Verification items for the finished model (mm, model axes). A direction names the side the tool comes from. Coordinates: 2 decimals unless noted, no trailing zeros. Write each loop counter-clockwise with the first axis right and the second up, starting at its lowest first coordinate (ties: lowest second). Pieces come first, ordered by that corner, then holes. Notation, with made-up numbers: (10.25, 7) -> (50.25, 7) arc R26 cw to (50.25, 39) -> close; hole circle Ø2 at (23, 50). An arc over 180 degrees is marked (long way). Answer in a Markdown table with one row per item.
```python
from build123d import *

# Parameters (mm, degrees)
SKETCH1_R           = 12.7
BOSS_EXTRUDE1_DEPTH = 3.81
EXTRUDE_THIN1_START = -3.81
EXTRUDE_THIN1_DEPTH = 7.62
EXTRUDE_THIN4_DEPTH = 3.81
SCALE1_SCALE        = 1.5


# Read off the part's stored shape, not the designer's step: Extrude-Thin1
with BuildPart() as part:
    # Sketch1 → Boss-Extrude1 (new, symmetric)
    with BuildSketch(Plane.XY):
        with Locations(Location((0, 0, 0), (0, 0, 180))):
            Circle(SKETCH1_R)
    extrude(amount=BOSS_EXTRUDE1_DEPTH, both=True)



with BuildPart() as body_2:
    # Extrude-Thin1 outline → Extrude-Thin1 (new body)
    with BuildSketch(Plane.XY.offset(EXTRUDE_THIN1_START)):
        Polygon((14.568006187, -139.326398763), (1.905, -76.011367827), (1.905, -12.7), (-1.905, -12.7), (-1.905, -76.011367827), (-14.568006187, -139.326398763), (-10.831993813, -140.073601237), (0, -85.913632173), (10.831993813, -140.073601237), align=None)
    extrude(amount=EXTRUDE_THIN1_DEPTH)


with BuildPart() as part_1:
    add(part.part)

    add(body_2.part)  # Extrude-Thin4 merges body 2
    # Sketch1<4> → Extrude-Thin4 (add, symmetric)
    with BuildSketch(Plane.XY):
        Polygon((13.945337458, -75.950932508), (0, -6.224245218), (-13.945337458, -75.950932508), (-11.454662542, -76.449067492), (0, -19.175754782), (11.454662542, -76.449067492), align=None)
    extrude(amount=EXTRUDE_THIN4_DEPTH, both=True)


with BuildPart() as part_2:
    # Scale1: scaled about (0, -50.73447441, 0)
    add(part_1.part.scale(SCALE1_SCALE).moved(Location((0, 25.367237205, 0))))


solid = part_2.part
```
1. Thickness scan on line 1 (X direction, y = -24, z = 1.75); line 2 (X direction, y = -84, z = -1.25); line 3 (X direction, y = -161, z = 4). Record the ranges inside material, lowest first. Write a range as from..to.
Geometry says:
| item | result |
|---|---|
| line 1 | -8.01..-4.12, -2.86..2.86, 4.12..8.01 |
| line 2 | -20.01..-16.12, -2.86..2.86, 16.12..20.01 |
| line 3 | -17.33..-11.5, 11.5..17.33 |
2. Section check A-A, the plane y = -167.5. Record the boundary of the cut face in (x, z) (3 decimals).
Geometry says:
| item | result |
|---|---|
| outline | (-18.628, -5.715) -> (-12.799, -5.715) -> (-12.799, 5.715) -> (-18.628, 5.715) -> close; (12.799, -5.715) -> (18.628, -5.715) -> (18.628, 5.715) -> (12.799, 5.715) -> close |
3. Section check C-C, the plane z = 4. Record the boundary of the cut face in (x, y), plus the area to 3 significant figures.
Geometry says:
| item | result |
|---|---|
| outline | (-21.85, -183.62) -> (-16.25, -184.74) -> (0, -103.5) -> (16.25, -184.74) -> (21.85, -183.62) -> (2.86, -88.65) -> (2.86, -17.68) -> (17.18, -89.31) -> (20.92, -88.56) -> (2.86, 1.74) -> (2.86, 6.32) -> (1.94, 6.32) -> (1.92, 6.41) arc R19.05 ccw (long way) to (-1.92, 6.41) -> (-1.94, 6.32) -> (-2.86, 6.32) -> (-2.86, 1.74) -> (-20.92, -88.56) -> (-17.18, -89.31) -> (-2.86, -17.68) -> (-2.86, -88.65) -> close |
| area | 3,380 mm^2 |
4. Section check B-B, the plane x = -5. Record the boundary of the cut face in (y, z) (3 decimals), plus the area to 3 significant figures.
Geometry says:
| item | result |
|---|---|
| outline | (-128.503, -5.715) -> (-99.362, -5.715) -> (-99.362, 5.715) -> (-128.503, 5.715) -> close; (-28.396, -5.715) -> (-8.969, -5.715) -> (-8.969, 5.715) -> (-28.396, 5.715) -> close; (6.985, -5.715) -> (43.749, -5.715) -> (43.749, 5.715) -> (6.985, 5.715) -> close |
| area | 975 mm^2 |
5. Section check D-D, the plane y = 17.5. Record the boundary of the cut face in (x, z) (3 decimals).
Geometry says:
| item | result |
|---|---|
| outline | (-17.35, -5.715) -> (17.35, -5.715) -> (17.35, 5.715) -> (-17.35, 5.715) -> close |
6. Tool access check on faces 5 (the flat face through (-8.238, -144.692, -0.08)), 6 (the flat face through (-10.12, -54, 0.08)), 7 (the flat face through (-19.076, -88.928, 0.08)). Record the directions out of +Z, -Z, +X, -X, +Y, -Y that give a thin tool (end or side, any length) a straight path to the whole face; none if there is none.
Geometry says:
| item | result |
|---|---|
| face 5 | +Z, -Z, -Y |
| face 6 | +Z, -Z |
| face 7 | +Z, -Z, -X |
7. Mould release check, pull along X, two halves, no side actions. Record for faces 1 (the flat face through (-19.089, -184.175, -0.08)), 2 (the flat face through (8.01, -143.55, -0.08)), 3 (the flat face through (2.858, -54, 0)), 4 (the flat face through (12.014, -44.04, 0.08)): released by +X, released by -X, zero draft, split by the parting line, or undercut.
Geometry says:
| item | result |
|---|---|
| face 1 | released by -X |
| face 2 | undercut |
| face 3 | undercut |
| face 4 | released by +X |
8. Depth check by flat-ended pin: P1, Ø4, axis at y = -112, z = 3.5, coming from the -X side; P2, Ø0.5, axis at x = -2, z = 2, coming from the +Y side; P3, Ø4, axis at x = -16.5, z = 3.5, coming from the +Y side; P4, Ø5, axis at x = 6.5, y = -58, coming from the -Z side. Enter the tip coordinate at first touch or a pass-through.
Geometry says:
| item | result |
|---|---|
| P1 | x = -7.93 |
| P2 | y = 44.34 |
| P3 | y = 37.72 |
| P4 | through |
